Here's the drawing with two shaded views (mm, measured from the low corner). I have some questions. Coordinates: 2 decimals unless noted, no trailing zeros. Loops run counter-clockwise (first coordinate to the right, second up) from the corner with the lowest first, then second, coordinate; pieces in that order, holes last. Notation, with made-up numbers: (21, -8) -> (54, -8) arc R27 ccw to (54, 22) -> close; hole circle Ø11 at (12, 66.25). An arc over 180 degrees is marked (long way). Answer as a JSON object with one key per item and string values. Group by question number.
1) I want a section at C-C (y = 26). Write out the boundary of the cut face in (x, z), then the cut area to 3 significant figures.
2) If we mould it in two halves opening along Z, with no side actions, what happens to the marked faces 1, 2 and 3? For each: +Z half, -Z half, draft (parallel to the pull), parting line (faces both ways), or undercut.
3) I'm going to push flat-ended pins straight in: pin 1 (10 mm diameter, centred on x = 22, y = 15.5, fed in from -Z); pin 2 (6 mm diameter, centred on x = 32, y = 111, fed in from -Z); pin 3 (3 mm diameter, centred on x = 22.5, y = 114, fed in from -Z); pin 4 (10 mm diameter, centred on y = 95, z = 40.5, fed in from -X). Where does each tip first touch, or does it pass through?
4) I want a section at B-B (y = 72.5). Write out the boundary of the cut face in (x, z).
5) I need wall thicknesses on probe 1 along Z at (x, y) = (40, 121); probe 2 along Y at (x, z) = (55, 5); probe 3 along X at (y, z) = (28, 28). Which ranges of each line are inside material? Lowest first, please. Write a range as [from, to].
6) I want a section at A-A (y = 119.5). Write out the boundary of the cut face in (x, z).
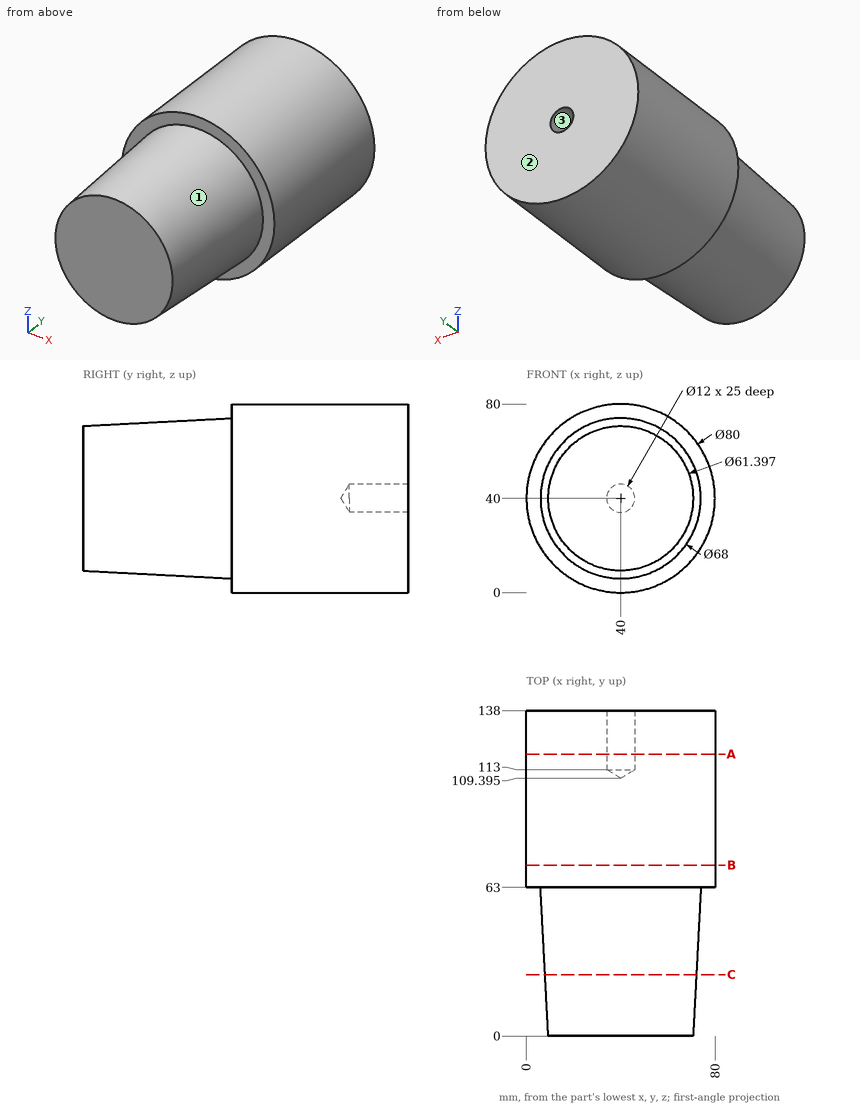
Determined:
{
 "1": {"outline": "circle Ø64.12 at (40, 40)", "area": "3,230 mm^2"},
 "2": {"face 1": "parting line", "face 2": "draft", "face 3": "undercut"},
 "3": {"pin 1": "z = 11.28", "pin 2": "z = 0.31", "pin 3": "z = 3.34", "pin 4": "x = 0"},
 "4": {"outline": "circle Ø80 at (40, 40)"},
 "5": {"probe 1": "[0, 34], [46, 80]", "probe 2": "[63, 138]", "probe 3": "[10.16, 69.84]"},
 "6": {"outline": "circle Ø80 at (40, 40); hole circle Ø12 at (40, 40)"}
}
